from build123d import *

# Parameters (mm, degrees)
BOSS_EXTRUDE1_DEPTH = 12
SKETCH2_R           = 8
CUT_EXTRUDE1_DEPTH  = 56.172456897
SKETCH3_R           = 8
BOSS_EXTRUDE2_DEPTH = 12
BOSS_EXTRUDE3_START = -12
SKETCH4_R           = 8
BOSS_EXTRUDE3_DEPTH = 12
SKETCH5_R           = 8
BOSS_EXTRUDE4_DEPTH = 12
FILLET1_R           = 2


with BuildPart() as part:
    # Sketch1 → Boss-Extrude1 (new body)
    with BuildSketch(Plane(origin=(0, 0, 0), x_dir=(1, 0, 0), z_dir=(0, 1, 0))):
        with BuildLine():
            Line((-30, 20), (-30, -20))
            Line((-30, -20), (30, -20))
            ThreePointArc((30, -20), (50, 0), (30, 20))
            Line((30, 20), (-30, 20))
        make_face()
    extrude(amount=BOSS_EXTRUDE1_DEPTH)

    # Sketch2 → Cut-Extrude1 (cut, through all)
    with BuildSketch(Plane(origin=(0, 12, 0), x_dir=(1, 0, 0), z_dir=(0, 1, 0))):
        with Locations(Location((30, 0, 0), (0, 0, 270))):
            Circle(SKETCH2_R)
    extrude(amount=-CUT_EXTRUDE1_DEPTH, mode=Mode.SUBTRACT)

    # Sketch3 → Boss-Extrude2 (add)
    with BuildSketch(Plane.XY.offset(20)):
        with BuildLine():
            Line((-30, 32), (-30, 12))
            Line((-30, 12), (10, 12))
            Line((10, 12), (10, 32))
            ThreePointArc((10, 32), (-10, 52), (-30, 32))
        make_face()
        with Locations((-10, 32)):
            Circle(SKETCH3_R, mode=Mode.SUBTRACT)
    extrude(amount=-BOSS_EXTRUDE2_DEPTH)

    # Sketch4 → Boss-Extrude3 (add)
    with BuildSketch(Plane(origin=(0, 0, -20), x_dir=(-1, 0, 0), z_dir=(0, 0, -1)).offset(BOSS_EXTRUDE3_START)):
        with BuildLine():
            Line((-10, 32), (-10, 12))
            Line((-10, 12), (30, 12))
            Line((30, 12), (30, 32))
            ThreePointArc((30, 32), (10, 52), (-10, 32))
        make_face()
        with Locations(Location((10, 32, 0), (0, 0, 180))):
            Circle(SKETCH4_R, mode=Mode.SUBTRACT)
    extrude(amount=BOSS_EXTRUDE3_DEPTH)

    # Sketch5 → Boss-Extrude4 (add)
    with BuildSketch(Plane.ZY.offset(30)):
        with BuildLine():
            Line((-20, -20), (-20, 0))
            Line((-20, 0), (20, 0))
            Line((20, 0), (20, -20))
            ThreePointArc((20, -20), (0, -40), (-20, -20))
        make_face()
        with Locations((0, -20)):
            Circle(SKETCH5_R, mode=Mode.SUBTRACT)
    extrude(amount=-BOSS_EXTRUDE4_DEPTH)

    # Fillet1
    fillet1_edges = [part.edges().sort_by_distance(p)[0] for p in [
        (-10, 12, 8),
        (10, 12, 14),
        (-10, 12, -8),
        (10, 12, -14),
        (-18, 0, 0),
    ]]
    fillet(fillet1_edges, radius=FILLET1_R)


solid = part.part
For this review, take the finished solid that the model builds, in its own axes (mm). A direction names the side the tool comes from. Coordinates: 2 decimals unless noted, no trailing zeros. Order: outer loops, then holes, each group sorted by start corner. A loop starts at its lowest first (then second) coordinate and runs counter-clockwise, first axis right, second up. Notation, with made-up numbers: (-15.5, 53) -> (25.5, 53) arc R24 cw to (25.5, 65) -> close; hole circle Ø3 at (-16, 56.5). An arc over 180 degrees is marked (long way). Return JSON: item names as keys, results as strings.
1. We need section A-A on z = 12. Write out the cut boundary in (x, y), and give its area (3 significant figures).
Answer block:
{"outline": "(-30, -36) -> (-18, -36) -> (-18, -2) arc R2 cw to (-16, 0) -> (46, 0) -> (46, 12) -> (12, 12) arc R2 cw to (10, 14) -> (10, 32) arc R20 ccw to (-30, 32) -> close; hole circle Ø16 at (-10, 32)", "area": "2,570 mm²"}
2. We need section D-D on x = 24.5. Write out the cut boundary in (y, z), and give its area (3 significant figures).
Answer block:
{"outline": "(0, -20) -> (12, -20) -> (12, -5.81) -> (0, -5.81) -> close; (0, 5.81) -> (12, 5.81) -> (12, 20) -> (0, 20) -> close", "area": "341 mm²"}
3. For pin 1 Ø9.5 at (y, z) = (-20, 0) entering from -X; pin 2 Ø3 at (x, z) = (36.5, -15) entering from +Y; pin 3 Ø11.5 at (y, z) = (-23, 6.5) entering from +X; pin 4 Ø3 at (x, z) = (4.5, 7.5) entering from +Y, all flat-tipped, find the tip position at first contact; note any pin that passes through.
Answer block:
{"pin 1": "through", "pin 2": "y = 12", "pin 3": "x = -18", "pin 4": "y = 47.12"}
4. Machinability: for faces 1 (the cylindrical face through (-9.29, 12.6, -7.43)), 2 (the flat face through (17, 0, 0)), 3 (the flat face through (10, 23, 14)), which of the approach directions +Z, -Z, +X, -X, +Y, -Y give a long, thin tool a straight path to every point of the face, cutting with its end or side? Answer none if there is none.
Answer block:
{"face 1": "+X, -X, +Y", "face 2": "+Z, -Z, +X, -Y", "face 3": "+Z, -Z, +X, +Y"}
5. We need section B-B on x = -10. Write out the cut boundary in (y, z), and give its area (3 significant figures).
Answer block:
{"outline": "(0, -20) -> (24, -20) -> (24, -8) -> (14, -8) arc R2 cw to (12, -6) -> (12, 6) arc R2 cw to (14, 8) -> (24, 8) -> (24, 20) -> (0, 20) -> close; (40, -20) -> (52, -20) -> (52, -8) -> (40, -8) -> close; (40, 8) -> (52, 8) -> (52, 20) -> (40, 20) -> close", "area": "1,060 mm²"}
6. For line 1 (X direction, y = 32, z = -11.25); line 2 (Z direction, x = -12, y = 47); line 3 (Y direction, x = -24, z = 0), list the stretches that pass through material, from the lowest coordinate up. Write a range as from..to.
Answer block:
{"line 1": "-30..-18, -2..10", "line 2": "-20..-8, 8..20", "line 3": "-40..-28, -12..12"}
7. We need section C-C on z = 0. Write out the cut boundary in (x, y), and give its area (3 significant figures).
Answer block:
{"outline": "(-30, -40) -> (-18, -40) -> (-18, -28) -> (-30, -28) -> close; (-30, -12) -> (-18, -12) -> (-18, -2) arc R2 cw to (-16, 0) -> (22, 0) -> (22, 12) -> (-30, 12) -> close; (38, 0) -> (50, 0) -> (50, 12) -> (38, 12) -> close", "area": "1,060 mm²"}
8. The part is to be moulded in two halves that separate along Z. For faces 4 (the cylindrical face through (50, 6, 0)), 5 (the flat face through (-18, -12, -4)), 6 (the cylindrical face through (-24.08, -27.81, -1.73)), say which applies: +Z half, -Z half, draft (parallel to the pull), parting line (faces both ways), or undercut.
Answer block:
{"face 4": "parting line", "face 5": "draft", "face 6": "undercut"}
